Autodesk Inventor part; units mm, degrees
ref_plane "YZ Plane" through (0, 0, 0) normal (1, 0, 0) x (0, 1, 0)
ref_plane "XZ Plane" through (0, 0, 0) normal (0, 1, 0) x (-1, 0, 0)
ref_plane "XY Plane" through (0, 0, 0) normal (0, 0, 1) x (1, 0, 0)
sketch "Sketch1" plane through (0, 0, 0) normal (0, 1, 0) x (-1, 0, 0)
  line L0 (0, -62.5) -> (0, 62.5) construction
  line L1 (-4.45, 66.95) -> (-4.45, 58.05)
  line L2 (-4.45, 58.05) -> (14.5, 58.05)
  line L3 (14.5, 58.05) -> (14.5, -58.05)
  line L4 (14.5, -58.05) -> (-4.45, -58.05)
  line L5 (-4.45, -58.05) -> (-4.45, -66.95)
  line L6 (-4.45, -66.95) -> (28.4, -66.95)
  line L7 (28.4, -66.95) -> (28.4, 66.95)
  line L8 (28.4, 66.95) -> (-4.45, 66.95)
  line L9 (0, 62.5) -> (-4.45, 62.5) construction
  line L10 (-4.45, -62.5) -> (0, -62.5) construction
  point P0 (0, 0)
  point P1 (0, 0)
  dimension "d0" = 125
  dimension "d1" = 4.45
  dimension "d2" = 4.45
  dimension "d3" = 13.9
  dimension "d4" = 14.5
  dimension "d5" = 4.45
extrude "Extrusion1" add sketch "Sketch1" along normal blind 3
hole "Hole1" at (0, 0, 62.5) at (0, 0, -62.5) direction (0, 1, 0) diameter 5 end through all
fillet "Fillet1" radius 1.5 8 edges at (-14.5, 1.5, 58.05) (-28.4, 1.5, 66.95) (-14.5, 1.5, -58.05) (-28.4, 1.5, -66.95) (4.45, 1.5, -58.05) (4.45, 1.5, -66.95) (4.45, 1.5, 58.05) (4.45, 1.5, 66.95)
sketch "Sketch2" plane through (0, 3, 0) normal (0, 1, 0) x (1, 0, 0)
  arc A0 (-26.9, 66.95) -> (-28.4, 65.45) centre (-26.9, 65.45) ccw
  line L0 (-28.4, 65.45) -> (-28.4, -65.45)
  arc A1 (-28.4, -65.45) -> (-26.9, -66.95) centre (-26.9, -65.45) ccw
  line L1 (-26.9, -66.95) -> (2.95, -66.95)
  line L2 (4.45, -65.45) -> (4.45, -59.55)
  line L3 (2.95, -58.05) -> (-13, -58.05)
  arc A2 (-14.5, -56.55) -> (-13, -58.05) centre (-13, -56.55) ccw
  line L4 (-14.5, -56.55) -> (-14.5, 56.55)
  arc A3 (-13, 58.05) -> (-14.5, 56.55) centre (-13, 56.55) ccw
  line L5 (-13, 58.05) -> (2.95, 58.05)
  line L6 (4.45, 59.55) -> (4.45, 65.45)
  line L7 (2.95, 66.95) -> (-26.9, 66.95)
  circle A4 centre (0, -62.5) radius 2.5
  circle A5 centre (0, 62.5) radius 2.5
  line L8 (4.45, -65.45) -> (4.45, -59.55) construction
  line L9 (4.45, -62.5) -> (-28.4, -62.5) construction
  line L10 (-28.4, 65.45) -> (-28.4, -65.45) construction
  line L11 (4.45, 59.55) -> (4.45, 65.45) construction
  line L12 (4.45, 62.5) -> (-28.4, 62.5) construction
  line L13 (-14.5, 0) -> (-28.4, 0) construction
  line L14 (2.95, 66.95) -> (-26.9, 66.95) construction
  line L15 (-26.9, -66.95) -> (2.95, -66.95) construction
  line L16 (-23.95, 66.95) -> (-23.95, -66.95) construction
  arc A6 (2.95, -66.95) -> (4.45, -65.45) centre (2.95, -65.45) ccw
  arc A7 (4.45, -59.55) -> (2.95, -58.05) centre (2.95, -59.55) ccw
  arc A8 (2.95, 58.05) -> (4.45, 59.55) centre (2.95, 59.55) ccw
  arc A9 (4.45, 65.45) -> (2.95, 66.95) centre (2.95, 65.45) ccw
  point P0 (0, 0)
  point P1 (4.45, -66.95)
  point P2 (4.45, -58.05)
  point P3 (4.45, 58.05)
  point P4 (4.45, 66.95)
  point P5 (-21.45, 0)
  point P6 (-23.95, -62.5)
  point P7 (-16.45, -62.5)
  point P8 (-23.95, -55)
  point P9 (-23.95, 62.5)
  point P10 (-16.45, 62.5)
  point P11 (-23.95, 55)
  dimension "d7" = 0
  dimension "d17" = 7.5
  dimension "d25" = 4.45
  dimension "d26" = 7.5
hole "Hole2" at (-23.95, 3, 62.5) at (-16.45, 3, 62.5) at (-23.95, 3, 55) at (-23.95, 3, -55) at (-23.95, 3, -62.5) at (-16.45, 3, -62.5) direction (0, -1, 0) diameter 3 end through all
equation "\"d0\" = holes_spacing"
equation "\"d1\" = 0.5 * width"
equation "\"d2\" = 0.5 * width"
equation "\"d3\" = width + back_extra_width"
equation "\"d4\" = holes_2_back"
equation "\"d5\" = 0.5 * width"
equation "\"d6\" = thickness"
equation "\"d25\" = 0.5 * width"
equation "\"thickness\" = 3"
equation "\"holes_spacing\" = 125"
equation "\"holes_2_back\" = 14.5"
equation "\"width\" = 8.9"
equation "\"piano_wire_holes_spacing\" = 7.5"
equation "\"back_extra_width\" = 5"
properties part number "nuc_fix_v2"
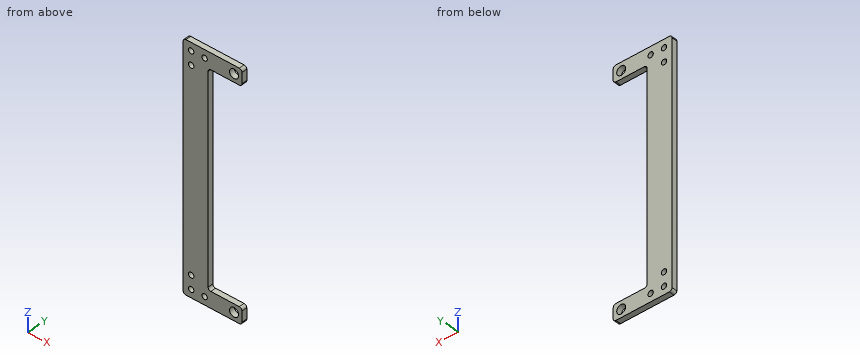
The listing builds one solid part. Answer for the finished solid, in the listing's coordinates (mm). Coordinates: 2 decimals unless noted, no trailing zeros. Write each loop counter-clockwise with the first axis right and the second up, starting at its lowest first coordinate (ties: lowest second). Pieces come first, ordered by that corner, then holes. Notation, with made-up numbers: (-26, 40.5) - (-11, 40.5) arc R26 cw to (-11, 64.5) - close; hole circle Ø6 at (-25.75, 1). An arc over 180 degrees is marked (long way). Return JSON: item names as keys, results as strings. Group by question number.
Q1. The part is cut by section B-B on y = 2.1. State how many separate pieces and enclosed holes the cut face has, and give its area (3 significant figures).
Q2. The part is cut by section C-C on x = -23.95. Write down the section's boundary in (y, z).
Q3. The part is cut by section A-A on z = -55. Write down the section's boundary in (x, y), and give its area (3 significant figures).
Q4. Flat-ended cylindrical pins translate along their axes: pin 1 Ø2.5 at (x, z) = (-16.45, -62.5) entering from -Y; pin 2 Ø1.5 at (x, z) = (-17, 6.5) entering from -Y; pin 3 Ø0.9 at (y, z) = (1, 6) entering from +X. Find the tip coordinate at first contact, or state that the pin passes through.
Q5. Find the intervals of material crossed by line 1 along Z through (x, y) = (-23.95, 1.35); line 2 along Z through (x, y) = (0, 1.75); line 3 along X through (y, z) = (1.7, -62.5), in increasing order. Write a range as [from, to].
Q6. The part is cut by section D-D on x = 0. Write down the section's boundary in (y, z).
Evaluation:
{
 "1": {"separate pieces": "1", "enclosed holes": "8", "area": "2,110 mm2"},
 "2": {"outline": "(0, -66.95) - (3, -66.95) - (3, -64) - (0, -64) - close; (0, -61) - (3, -61) - (3, -56.5) - (0, -56.5) - close; (0, -53.5) - (3, -53.5) - (3, 53.5) - (0, 53.5) - close; (0, 56.5) - (3, 56.5) - (3, 61) - (0, 61) - close; (0, 64) - (3, 64) - (3, 66.95) - (0, 66.95) - close"},
 "3": {"outline": "(-28.4, 0) - (-25.45, 0) - (-25.45, 3) - (-28.4, 3) - close; (-22.45, 0) - (-14.5, 0) - (-14.5, 3) - (-22.45, 3) - close", "area": "32.7 mm2"},
 "4": {"pin 1": "passes through", "pin 2": "stops at y = 0", "pin 3": "stops at x = -14.5"},
 "5": {"line 1": "z = [-66.95, -64], [-61, -56.5], [-53.5, 53.5], [56.5, 61], [64, 66.95]", "line 2": "z = [-66.95, -65], [-60, -58.05], [58.05, 60], [65, 66.95]", "line 3": "x = [-28.4, -25.45], [-22.45, -17.95], [-14.95, -2.5], [2.5, 4.45]"},
 "6": {"outline": "(0, -66.95) - (3, -66.95) - (3, -65) - (0, -65) - close; (0, -60) - (3, -60) - (3, -58.05) - (0, -58.05) - close; (0, 58.05) - (3, 58.05) - (3, 60) - (0, 60) - close; (0, 65) - (3, 65) - (3, 66.95) - (0, 66.95) - close"}
}
